For this review, take the finished solid that the model builds, in its own axes (mm). Face numbers are marked on the shaded views. Coordinates: 2 decimals unless noted, no trailing zeros. Loops run counter-clockwise (first coordinate to the right, second up) from the corner with the lowest first, then second, coordinate; pieces in that order, holes last.
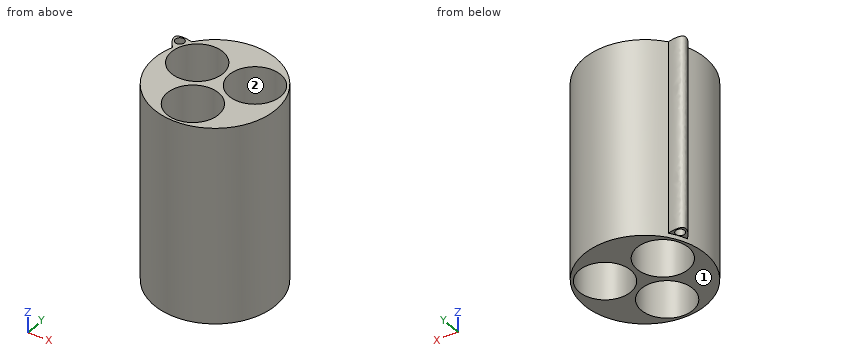
```python
from build123d import *

# Parameters (mm, degrees)
SKETCH1_R           = 21.59
SKETCH1_R_2         = 9.144
BOSS_EXTRUDE1_DEPTH = 70.1
SKETCH2_R           = 1.5875
BOSS_EXTRUDE3_DEPTH = 68.58


with BuildPart() as part:
    # Sketch1 → Boss-Extrude1 (new body)
    with BuildSketch(Plane.XY):
        Circle(SKETCH1_R)
        with Locations((0.118855304, -11.557)):
            Circle(SKETCH1_R_2, mode=Mode.SUBTRACT)
        with Locations((9.955579479, 5.869470694)):
            Circle(SKETCH1_R_2, mode=Mode.SUBTRACT)
        with Locations((-10.060900468, 5.687049391)):
            Circle(SKETCH1_R_2, mode=Mode.SUBTRACT)
    extrude(amount=BOSS_EXTRUDE1_DEPTH)

    # Sketch2 → Boss-Extrude3 (add)
    with BuildSketch(Plane.XY.offset(70.1)):
        with BuildLine():
            ThreePointArc((-20.134392286, 7.793224446), (-18.801139076, 10.613447577), (-17.075379878, 13.212096806))
            add(Edge.make_bspline(
                [(-20.134392286, 7.793224446), (-26.24429958, 15.203378156), (-17.075379878, 13.212096806)],
                knots=[0, 0, 0, 1, 1, 1], degree=2))
        make_face()
        with Locations((-20.134392286, 11.624596806)):
            Circle(SKETCH2_R, mode=Mode.SUBTRACT)
    extrude(amount=-BOSS_EXTRUDE3_DEPTH)


solid = part.part
```
Q1. For pin 1 Ø3 at (x, z) = (4, 19.5) entering from +Y; pin 2 Ø12 at (y, z) = (-1, 21) entering from -X; pin 3 Ø4 at (y, z) = (6, 18) entering from +X, all flat-tipped, find the tip position at first contact; note any pin that passes through.
Q2. Consider section B-B (y = 0). State the section outline as (x, z) points.
Q3. Consider section D-D (x = -2.5). State the section outline as (y, z) points, then the cut area to 3 significant figures.
Q4. Consider section A-A (x = -12). State the section outline as (y, z) points.
Q5. The part is to be moulded in two halves that separate along Y. For the marked faces 1 and 2, say which applies: +Y half, -Y half, draft (parallel to the pull), parting line (faces both ways), or undercut.
Q6. Consider section C-C (y = -6.5). State the section outline as (x, z) points.
Q7. Wall thickness on probe 1 along X at (y, z) = (1, 24); probe 2 along X at (y, z) = (3, 31.5); probe 3 along Y at (x, z) = (-7, 12): over which ranges is each line inside the solid? List them lowest first.
Model answer:
1. pin 1: stops at y = 21.44
1. pin 2: stops at x = -21.59
1. pin 3: stops at x = 21.22
2. outline: (-21.59, 0) - (-17.22, 0) - (-17.22, 70.1) - (-21.59, 70.1) - close; (-2.9, 0) - (2.94, 0) - (2.94, 70.1) - (-2.9, 70.1) - close; (16.97, 0) - (21.59, 0) - (21.59, 70.1) - (16.97, 70.1) - close
3. outline: (-21.44, 0) - (-20.32, 0) - (-20.32, 70.1) - (-21.44, 70.1) - close; (-2.8, 0) - (0.54, 0) - (0.54, 70.1) - (-2.8, 70.1) - close; (10.83, 0) - (21.44, 0) - (21.44, 70.1) - (10.83, 70.1) - close
3. area: 1,060 mm2
4. outline: (-17.95, 0) - (-3.25, 0) - (-3.25, 70.1) - (-17.95, 70.1) - close; (14.62, 0) - (17.95, 0) - (17.95, 70.1) - (14.62, 70.1) - close
5. face 1: draft
5. face 2: undercut
6. outline: (-20.59, 0) - (-7.5, 0) - (-7.5, 70.1) - (-20.59, 70.1) - close; (7.74, 0) - (20.59, 0) - (20.59, 70.1) - (7.74, 70.1) - close
7. probe 1: x = -21.57 to -17.91, -2.21 to 2.22, 17.7 to 21.57
7. probe 2: x = -21.38 to -18.8, -1.32 to 1.27, 18.64 to 21.38
7. probe 3: y = -20.42 to -17.3, -5.82 to -2.93, 14.3 to 20.42
